Build history of the part. All positions in model axes, mm. A direction names the side the tool comes from. Give positions to 0.01 mm unless a question says otherwise; leave off trailing zeros. Write each loop counter-clockwise with the first axis right and the second up, starting at its lowest first coordinate (ties: lowest second). Pieces come first, ordered by that corner, then holes. Notation, with made-up numbers: (64, 3.5) -> (88, 3.5) arc R16 cw to (88, 10.5) -> close; hole circle Ø6 at (19.5, 67). An arc over 180 degrees is marked (long way). One line per question, with ' | ' between items. Start each with the question number.
(1) Pull direction X, two halves, no side cores. Call faces 1 (the flat face through (134.72, 12, 8)), 2 (the cylindrical face through (142.79, 31.86, 6.59)), 3 (the cylindrical face through (-8, 31.93, 6.59)): released by +X, released by -X, zero draft, split by the parting line, or undercut.
(2) Drill centre lines: probe 1 along Y at (x, z) = (-4.5, 2.15); probe 2 along Y at (x, z) = (-4.5, 9); probe 3 along Y at (x, z) = (139.22, 6.5). Where is each one in solid material? Low to high. Write a range as from..to.
(3) Band-saw the part on A-A, the plane z = 10.25. Give the cut face in (x, y), and give its area (3 significant figures).
(4) Tool access for faces 4 (the flat face through (68, 33.36, 6)), 5 (the flat face through (-5, 2.732, 9)), 6 (the flat face through (66, 0, 8)), 7 (the cylindrical face through (136.223, 28.228, 1.528)): list every direction of +Z, -Z, +X, -X, +Y, -Y with a clear straight run to the whole face (end or side of a thin tool).
(5) Pin check, flat tips, straight feed: P1, Ø3, axis at x = -4.5, y = 15.5, coming from the +Z side; P2, Ø4, axis at x = 89.5, y = 3, coming from the +Z side; P3, Ø3, axis at x = 140.5, y = -5, coming from the -Z side. Stop position of each tip, or through.
(6) Band-saw the part on B-B, the plane x = 54. Give the cut face in (y, z).
(7) Band-saw the part on C-C, the plane y = 10. Give the cut face in (x, z).
Autodesk Fusion 360 part; units mm, degrees
sketch "Sketch1" plane through (0, 0, 0) normal (0, 0, 1) x (1, 0, 0) in component "WeCopy"
  line L0 (0, 0) -> (134.72, 0)
  line L1 (134.72, 0) -> (134.72, 23.86)
  line L2 (134.72, 23.86) -> (0, 23.86)
  line L3 (0, 23.86) -> (0, 0)
  line L4 (-9.5, -9.5) -> (144.22, -9.5)
  line L5 (144.22, -9.5) -> (144.22, 33.36)
  line L6 (144.22, 33.36) -> (-9.5, 33.36)
  line L7 (-9.5, 33.36) -> (-9.5, -9.5)
  circle A0 centre (139.22, 28.36) radius 1.7
  circle A1 centre (139.22, -4.5) radius 1.7
  circle A2 centre (-4.5, 28.36) radius 1.7
  circle A3 centre (-4.5, -4.5) radius 1.7
  circle A4 centre (139.22, 28.36) radius 3
  circle A5 centre (139.22, -4.5) radius 3
  circle A6 centre (-4.5, -4.5) radius 3
  circle A7 centre (-4.5, 28.36) radius 3
  dimension "d1" = 134.72
  dimension "d2" = 23.86
  dimension "d3" = 153.72
  dimension "d4" = 42.86
  dimension "d5" = 9.5
  dimension "d6" = 9.5
  dimension "d7" = 9.5
  dimension "d8" = 9.5
  dimension "d9" = 3.4
  dimension "d10" = 3.4
  dimension "d11" = 3.4
  dimension "d12" = 3.4
  dimension "d13" = 5
  dimension "d14" = 5
  dimension "d15" = 5
  dimension "d16" = 5
  dimension "d17" = 5
  dimension "d18" = 5
  dimension "d19" = 5
  dimension "d20" = 5
  dimension "d21" = 6
  dimension "d22" = 6
  dimension "d23" = 6
  dimension "d24" = 6
extrude "Extrude2" add sketch "Sketch1" along normal blind 9.9 from surface at 3.1 contours A4 | A5 | A6 | A7 makes body 1 at (138.2645, 25.5162, 9.7) makes body 2 at (-1.5037, -4.6495, 9.7) makes body 3 at (142.2163, -4.6495, 9.7) makes body 4 at (-1.5037, 28.2105, 9.7) in component "WeCopy"
extrude "Extrude3" add sketch "Sketch1" along normal blind 13 contours L4 L5 L6 L7 bodies 1 2 3 4 in component "WeCopy"
extrude "Extrude4" add sketch "Sketch1" along normal blind 3 contours L0 L1 L2 L3 bodies 1 in component "WeCopy"
sketch "Sketch2" plane through (0, 0, 3) normal (0, 0, 1) x (-1, 0, 0) in component "WeCopy"
  line L0 (0, -23.86) -> (0, 0)
  line L1 (0, 0) -> (-134.72, 0)
  line L2 (-134.72, 0) -> (-134.72, -23.86)
  line L3 (-134.72, -23.86) -> (0, -23.86)
  line L4 (14, -21.2325) -> (-4.5, -21.2325)
  line L5 (-4.5, -21.2325) -> (-4.5, -2.7325)
  line L6 (-4.5, -2.7325) -> (14, -2.7325)
  line L7 (14, -2.7325) -> (14, -21.2325)
  line L8 (9.5, 9.5) -> (-144.22, 9.5)
  dimension "d35" = 18.5
  dimension "d36" = 18.5
  dimension "d37" = 12.2325
extrude "Extrude5" cut sketch "Sketch2" against normal blind 7.5 from surface at 10 contours L0 L4 L6 L7 bodies 1 in component "WeCopy"
fillet "Fillet1" radius 5 1 edges at (-9.5, 33.36, 6.5) on bodies 1 in component "WeCopy"
fillet "Fillet2" radius 5 1 edges at (-9.5, -9.5, 6.5) on bodies 1 in component "WeCopy"
fillet "Fillet3" radius 5 1 edges at (144.22, -9.5, 6.5) on bodies 1 in component "WeCopy"
fillet "Fillet4" radius 5 1 edges at (144.22, 33.36, 6.5) on bodies 1 in component "WeCopy"
component "WeCopy" placed x (1, 0, 0) y (0, 1, 0) z (0, 0, 1) at (0, 0, 0)
equation "d1 = 96.620 mm + 38.1 mm"
equation "d3 = 115.620 mm + 38.1 mm"
Results:
1) face 1: undercut | face 2: released by +X | face 3: released by -X
2) probe 1: y = -9.5..-7.5, -1.5..25.36, 31.36..33.36 | probe 2: y = -9.5..-6.2, -2.8..2.73, 21.23..26.66, 30.06..33.36 | probe 3: y = -9.5..-6.2, -2.8..26.66, 30.06..33.36
3) outline: (-9.5, -4.5) arc R5 ccw to (-4.5, -9.5) -> (139.22, -9.5) arc R5 ccw to (144.22, -4.5) -> (144.22, 28.36) arc R5 ccw to (139.22, 33.36) -> (-4.5, 33.36) arc R5 ccw to (-9.5, 28.36) -> (-9.5, 21.23) -> (0, 21.23) -> (0, 23.86) -> (134.72, 23.86) -> (134.72, 0) -> (0, 0) -> (0, 2.73) -> (-9.5, 2.73) -> close; hole circle Ø3.4 at (-4.5, -4.5); hole circle Ø3.4 at (-4.5, 28.36); hole circle Ø3.4 at (139.22, -4.5); hole circle Ø3.4 at (139.22, 28.36) | area: 3,140 mm²
4) face 4: +Z, -Z, +X, -X, +Y | face 5: +Z, -X | face 6: +Z | face 7: -Z
5) P1: stops at z = 5.5 | P2: stops at z = 3 | P3: stops at z = 3.1
6) outline: (-9.5, 0) -> (33.36, 0) -> (33.36, 13) -> (23.86, 13) -> (23.86, 3) -> (0, 3) -> (0, 13) -> (-9.5, 13) -> close
7) outline: (-9.5, 0) -> (144.22, 0) -> (144.22, 13) -> (134.72, 13) -> (134.72, 3) -> (0, 3) -> (0, 5.5) -> (-9.5, 5.5) -> close
